Verification items for the finished model (mm, model axes). Face numbers are marked on the shaded views. Round coordinates to 2 decimals unless told otherwise and drop trailing zeros. Loops run counter-clockwise (first coordinate to the right, second up) from the corner with the lowest first, then second, coordinate; pieces in that order, holes last. Notation, with made-up numbers: M 49,89 L 95,89 A33 ccw 95,123 Z; hole C 3,63.25 d6. An arc over 180 degrees is marked long. Answer as CSV lines item,"result".
```python
from build123d import *

# Parameters (mm, degrees)
F3_DEPTH = 19.05


with BuildPart() as f1:
    # F0 (on Front) → F1 (revolve)
    with BuildSketch(Plane.XZ):
        with BuildLine():
            Line((7.874, -20.32), (7.874, 20.32))
            Line((7.874, 20.32), (6.223, 20.32))
            Line((6.223, 20.32), (6.223, 13.0673574546))
            Line((6.223, 13.0673574546), (6.223, 12.827))
            ThreePointArc((6.223, 12.827), (6.4089871939, 12.3779871939), (6.858, 12.192))
            Line((6.858, 12.192), (6.858, -20.32))
            Line((6.858, -20.32), (7.874, -20.32))
        make_face()
    revolve(axis=Axis((0, 0, -2.1967927045), (0, 0, -1)))

    # F2 (on Top) → F3 (join, symmetric)
    with BuildSketch(Plane.XY):
        with BuildLine():
            Line((0.8456389311, -2.2599698667), (-6.1631355014, -3.0079768601))
            ThreePointArc((-6.1631355014, -3.0079768601), (-6.0475003842, -3.2341773457), (-5.9235668092, -3.4559398515))
            Line((-5.9235668092, -3.4559398515), (0.8995487584, -2.7651012659))
            Line((0.8995487584, -2.7651012659), (0.8456389311, -2.2599698667))
        make_face()
        with BuildLine():
            ThreePointArc((5.6865521256, -3.8334434812), (5.8246299338, -3.6202002893), (5.9547151099, -3.401989412))
            Line((5.9547151099, -3.401989412), (1.9448735611, 2.1615827097))
            Line((1.9448735611, 2.1615827097), (1.5343718508, 1.8623297301))
            Line((1.5343718508, 1.8623297301), (5.6865521256, -3.8334434812))
        make_face()
        with BuildLine():
            Line((-2.3800107819, 0.3976401366), (0.4765833759, 6.8414203413))
            ThreePointArc((0.4765833759, 6.8414203413), (0.2228704504, 6.8543776349), (-0.0311483008, 6.8579292635))
            Line((-0.0311483008, 6.8579292635), (-2.8444223195, 0.6035185562))
            Line((-2.8444223195, 0.6035185562), (-2.3800107819, 0.3976401366))
        make_face()
    extrude(amount=F3_DEPTH, both=True)

    # F4 (on Front) → F5 (revolve, cut)
    with BuildSketch(Plane.XZ):
        Polygon((0, -20.32), (6.858, -20.32), (6.858, -13.97), (0, -7.112), align=None)
        Polygon((0, 20.32), (0, 12.827), (0, 6.604), (6.223, 12.827), (6.223, 20.32), align=None)
    revolve(axis=Axis((0, 0, -2.1967927045), (0, 0, -1)), mode=Mode.SUBTRACT)


solid = f1.part
```
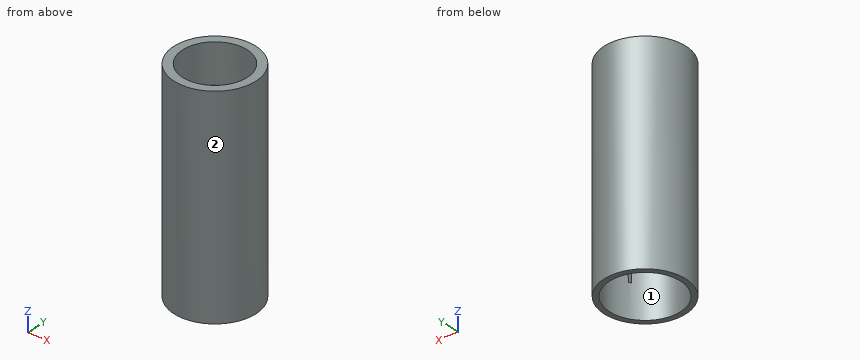
1) Go/stop test with flat-tipped pins: pin 1 (4 mm diameter, centred on y = -6, z = -2.5, fed in from +X); pin 2 (5 mm diameter, centred on x = 3.5, z = 7, fed in from +Y). Record where each tip stops, or that it passes through.
Here are the results:
pin 1,"stops at x = 6.78"
pin 2,"stops at y = 7.81"
2) Section check A-A (y = 0). Record the cut outline in (x, z) (3 decimals), plus the area to 3 significant figures.
Here are the results:
outline,"M -7.874,-20.32 L -6.858,-20.32 L -6.858,12.192 A0.635 ccw -6.223,12.827 L -6.223,20.32 L -7.874,20.32 Z; M 2.892,-10.004 L 3.503,-10.615 L 3.503,10.107 L 2.892,9.496 Z; M 6.223,12.827 A0.635 ccw 6.858,12.192 L 6.858,-20.32 L 7.874,-20.32 L 7.874,20.32 L 6.223,20.32 Z"
area,"105 mm^2"
3) Material ranges on probe 1 along X at (y, z) = (0, 16.5); probe 2 along Y at (x, z) = (-3, 10); probe 3 along X at (y, z) = (6, -5.5), recorded low to high.
Here are the results:
probe 1,"x = -7.87 to -6.22, 6.22 to 7.87"
probe 2,"y = -7.28 to -6.17, -3.16 to -2.67, 6.17 to 7.28"
probe 3,"x = -5.1 to -3.32, -0.42 to 0.1, 3.32 to 5.1"
4) Section check C-C (x = -4.5). State how many separate pieces and enclosed holes the cut face has, plus the area to 3 significant figures.
Here are the results:
separate pieces,"3"
enclosed holes,"0"
area,"130 mm^2"
5) Draft check along X on the marked faces 1 and 2. Enter one of: +X half, -X half, draft (parallel to the pull), parting line (faces both ways), or undercut.
Here are the results:
face 1,"undercut"
face 2,"parting line"
6) Section check B-B (z = 8). Record the cut outline in (x, y), plus the area to 3 significant figures.
Here are the results:
outline,"C 0,0 d15.75; hole M -6.16,-3.01 L 0.85,-2.26 L 0.9,-2.77 L -5.92,-3.46 A6.86 ccw 5.69,-3.83 L 1.53,1.86 L 1.94,2.16 L 5.95,-3.4 A6.86 ccw 0.48,6.84 L -2.38,0.4 L -2.84,0.6 L -0.03,6.86 A6.86 ccw Z"
area,"57.2 mm^2"
